Design review of the part built by this model. Coordinates are the model's own, in mm. Coordinates: 2 decimals unless noted, no trailing zeros.
Q1. For L1, parallel to Z at x = -34.35, y = 2.5; L2, parallel to Z at x = -40, y = 0.8; L3, parallel to X at y = 0.7, z = 82.5, list the stretches that pass through material, from the lowest coordinate up.
Q2. For pin 1 Ø3.5 at (x, z) = (34.35, 82.07) entering from -Y; pin 2 Ø1.5 at (x, y) = (11, 1.5) entering from +Z, all flat-tipped, find the tip position at first contact; note any pin that passes through.
Q3. Take a section at A-A, the plane y = 2.35. State how many separate pieces and enclosed holes the cut face has, plus the area to 3 significant figures.
from build123d import *

# Parameters (mm, degrees)
SKETCH_1_R      = 1.5
SKETCH_1_R_2    = 1.75
SKETCH_1_W      = 30
SKETCH_1_H      = 27
EXTRUDE_1_DEPTH = 3.175


with BuildPart() as part:
    # 草图1 → 凸台-拉伸1 (new body)
    with BuildSketch(Plane(origin=(0, 0, 0), x_dir=(1, 0, 0), z_dir=(0, 1, 0))):
        with BuildLine():
            Line((-60, 29.195444573), (-60, -155.195444573))
            ThreePointArc((-60, -155.195444573), (0, -173), (60, -155.195444573))
            Line((60, -155.195444573), (60, 29.195444573))
            ThreePointArc((60, 29.195444573), (0, 47), (-60, 29.195444573))
        make_face()
        with Locations((-57, -150)):
            Circle(SKETCH_1_R, mode=Mode.SUBTRACT)
        with Locations((57, -150)):
            Circle(SKETCH_1_R, mode=Mode.SUBTRACT)
        with Locations((57, 24)):
            Circle(SKETCH_1_R, mode=Mode.SUBTRACT)
        with Locations((-57, 24)):
            Circle(SKETCH_1_R, mode=Mode.SUBTRACT)
        with Locations((-14, 29.95)):
            Circle(SKETCH_1_R, mode=Mode.SUBTRACT)
        with Locations((-14, 20.05)):
            Circle(SKETCH_1_R, mode=Mode.SUBTRACT)
        with Locations((34.2, 29.95)):
            Circle(SKETCH_1_R, mode=Mode.SUBTRACT)
        with Locations((34.2, 20.05)):
            Circle(SKETCH_1_R, mode=Mode.SUBTRACT)
        with Locations((-40, -63)):
            Circle(SKETCH_1_R_2, mode=Mode.SUBTRACT)
        with Locations((-40, -143)):
            Circle(SKETCH_1_R_2, mode=Mode.SUBTRACT)
        with Locations((40, -143)):
            Circle(SKETCH_1_R_2, mode=Mode.SUBTRACT)
        with Locations((40, -63)):
            Circle(SKETCH_1_R_2, mode=Mode.SUBTRACT)
        with Locations((-34.35, -82.074857642)):
            Circle(SKETCH_1_R, mode=Mode.SUBTRACT)
        with Locations((-34.35, -125.274857642)):
            Circle(SKETCH_1_R, mode=Mode.SUBTRACT)
        with Locations((34.35, -125.274857642)):
            Circle(SKETCH_1_R, mode=Mode.SUBTRACT)
        with Locations((34.35, -82.074857642)):
            Circle(SKETCH_1_R, mode=Mode.SUBTRACT)
        with Locations((-34.35, -30.974465683)):
            Circle(SKETCH_1_R, mode=Mode.SUBTRACT)
        with Locations((34.35, -30.974465683)):
            Circle(SKETCH_1_R, mode=Mode.SUBTRACT)
        with BuildLine():
            Line((-8.55, 35), (28.75, 35))
            ThreePointArc((28.75, 35), (29.810660172, 34.560660172), (30.25, 33.5))
            Line((30.25, 33.5), (30.25, 16.5))
            ThreePointArc((30.25, 16.5), (29.810660172, 15.439339828), (28.75, 15))
            Line((28.75, 15), (-8.55, 15))
            ThreePointArc((-8.55, 15), (-9.610660172, 15.439339828), (-10.05, 16.5))
            Line((-10.05, 16.5), (-10.05, 33.5))
            ThreePointArc((-10.05, 33.5), (-9.610660172, 34.560660172), (-8.55, 35))
        make_face(mode=Mode.SUBTRACT)
        with BuildLine():
            Line((-8, 41.359537153), (8, 41.359537153))
            ThreePointArc((8, 41.359537153), (9.5, 42.859537153), (8, 44.359537153))
            Line((8, 44.359537153), (-8, 44.359537153))
            ThreePointArc((-8, 44.359537153), (-9.5, 42.859537153), (-8, 41.359537153))
        make_face(mode=Mode.SUBTRACT)
        with BuildLine():
            Line((-8, -170.359537153), (8, -170.359537153))
            ThreePointArc((8, -170.359537153), (9.5, -168.859537153), (8, -167.359537153))
            Line((8, -167.359537153), (-8, -167.359537153))
            ThreePointArc((-8, -167.359537153), (-9.5, -168.859537153), (-8, -170.359537153))
        make_face(mode=Mode.SUBTRACT)
        with BuildLine():
            Line((-48.5, 19.95), (-48.5, 3.95))
            ThreePointArc((-48.5, 3.95), (-50, 2.45), (-51.5, 3.95))
            Line((-51.5, 3.95), (-51.5, 19.95))
            ThreePointArc((-51.5, 19.95), (-50, 21.45), (-48.5, 19.95))
        make_face(mode=Mode.SUBTRACT)
        with BuildLine():
            Line((51.5, 3.95), (51.5, 19.95))
            ThreePointArc((51.5, 19.95), (50, 21.45), (48.5, 19.95))
            Line((48.5, 19.95), (48.5, 3.95))
            ThreePointArc((48.5, 3.95), (50, 2.45), (51.5, 3.95))
        make_face(mode=Mode.SUBTRACT)
        with BuildLine():
            Line((48.5, -145.95), (48.5, -129.95))
            ThreePointArc((48.5, -129.95), (50, -128.45), (51.5, -129.95))
            Line((51.5, -129.95), (51.5, -145.95))
            ThreePointArc((51.5, -145.95), (50, -147.45), (48.5, -145.95))
        make_face(mode=Mode.SUBTRACT)
        with BuildLine():
            Line((-51.5, -129.95), (-51.5, -145.95))
            ThreePointArc((-51.5, -145.95), (-50, -147.45), (-48.5, -145.95))
            Line((-48.5, -145.95), (-48.5, -129.95))
            ThreePointArc((-48.5, -129.95), (-50, -128.45), (-51.5, -129.95))
        make_face(mode=Mode.SUBTRACT)
        with Locations((0, -3)):
            Rectangle(SKETCH_1_W, SKETCH_1_H, mode=Mode.SUBTRACT)
    extrude(amount=EXTRUDE_1_DEPTH)


solid = part.part
Responses:
1. L1: z = -41.5 to 29.47, 32.47 to 80.57, 83.57 to 123.77, 126.77 to 167.5
1. L2: z = -39.47 to 61.25, 64.75 to 141.25, 144.75 to 165.47
1. L3: x = -60 to -35.79, -32.91 to 32.91, 35.79 to 60
2. pin 1: stops at y = 0
2. pin 2: stops at z = 172.52
3. separate pieces: 1
3. enclosed holes: 26
3. area: 22,900 mm2
